Check sheet for the modelled part. Datum: model origin and axes. Units: mm. Face numbers are marked on the shaded views. A direction names the side the tool comes from. Round coordinates to 2 decimals unless told otherwise and drop trailing zeros. Order: outer loops, then holes, each group sorted by start corner. A loop starts at its lowest first (then second) coordinate and runs counter-clockwise, first axis right, second up. Notation, with made-up numbers: (24.25, 85.25) -> (63.25, 85.25) arc R12 cw to (63.25, 107.25) -> close; hole circle Ø6 at (32, 27.5). An arc over 180 degrees is marked (long way). Answer in a Markdown table with one row per item. Add a question column.
1. Sectioned sample at C-C, the plane x = 9.5. Record the boundary of the cut face in (y, z), then the cut area to 3 significant figures.
2. Depth check by flat-ended pin: P1, Ø0.8, axis at x = 13, z = 13, coming from the -Y side; P2, Ø0.5, axis at y = -13, z = 10, coming from the +X side; P3, Ø2.5, axis at x = -0.5, z = 10, coming from the +Y side. Enter the tip coordinate at first touch or a pass-through.
3. Draft check along Y on the marked faces 4, 5 and 6. Enter one of: +Y half, -Y half, draft (parallel to the pull), parting line (faces both ways), or undercut.
4. Sectioned sample at B-B, the plane y = 11.5. Record the boundary of the cut face in (x, z), then the cut area to 3 significant figures.
5. Material ranges on L1, parallel to X at y = 9, z = 17.5; L2, parallel to X at y = -5.5, z = 8.25; L3, parallel to X at y = 9.5, z = 11, recorded low to high. Write a range as from..to.
6. Sectioned sample at D-D, the plane x = 5. Record the boundary of the cut face in (y, z).
7. Access from +Z, -Z, +X, -X, +Y, -Y to the whole of each face (thin tool, end or side, straight path). Record for the marked faces 1, 2 and 3.
8. Sectioned sample at A-A, the plane x = 13. Record the boundary of the cut face in (y, z), then the cut area to 3 significant figures.
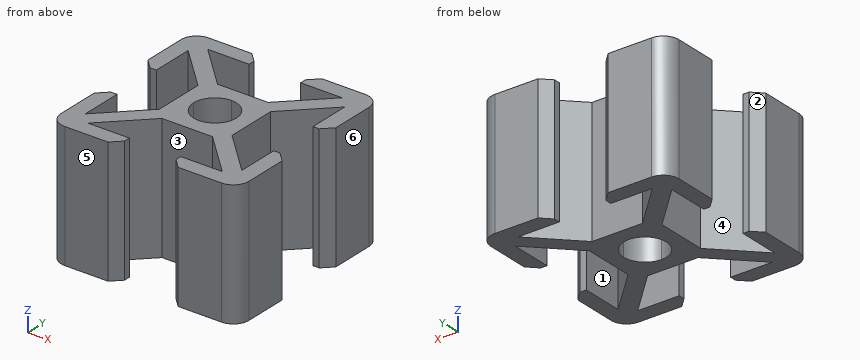
```python
from build123d import *

# Parameters (mm, degrees)
PAD_DEPTH            = 20
POLARPATTERN_COUNT   = 4
FILLET_R             = 2.5
CHAMFER_SIZE         = 1.5
BODY_PLACEMENT_ANGLE = 270


with BuildPart() as part:
    # Sketch → Pad (new body)
    with BuildSketch(Plane.XZ):
        with BuildLine():
            Line((0, 5.8), (4.032233, 5.8))
            Line((4.032233, 5.8), (10.732233, 12.5))
            Line((10.732233, 12.5), (4.1, 12.5))
            Line((4.1, 12.5), (4.1, 15))
            Line((4.1, 15), (15, 15))
            Line((15, 15), (15, 4.1))
            Line((15, 4.1), (12.5, 4.1))
            Line((12.5, 4.1), (12.5, 10.732233))
            Line((5.8, 4.032233), (12.5, 10.732233))
            Line((5.8, 4.032233), (5.8, 0))
            Line((3.4, 0), (5.8, 0))
            ThreePointArc((3.4, 0), (2.404163, 2.404163), (0, 3.4))
            Line((0, 5.8), (0, 3.4))
        make_face()
    pad = extrude(amount=PAD_DEPTH)

    # PolarPattern: Pad ×4 about axis
    polarpattern_axis = Axis((0, 0, 0), (0, -1, 0))
    for i in range(1, POLARPATTERN_COUNT):
        add(pad.rotate(polarpattern_axis, i * 360 / POLARPATTERN_COUNT))

    # Fillet
    fillet_edges = [part.edges().sort_by_distance(p)[0] for p in [
        (-15, -10, 15),
        (15, -10, 15),
        (15, -10, -15),
        (-15, -10, -15),
    ]]
    fillet(fillet_edges, radius=FILLET_R)

    # Chamfer
    chamfer_edges = [part.edges().sort_by_distance(p)[0] for p in [
        (4.1, -10, 15),
        (-4.1, -10, 15),
        (-15, -10, 4.1),
        (-15, -10, -4.1),
        (-4.1, -10, -15),
        (15, -10, -4.1),
        (4.1, -10, -15),
        (15, -10, 4.1),
    ]]
    chamfer(chamfer_edges, length=CHAMFER_SIZE)


with BuildPart() as part_1:
    # Body placement: moved
    add(part.part.rotate(Axis((0, 0, 0), (1, 0, 0)), BODY_PLACEMENT_ANGLE))


solid = part_1.part
```
Answer key:
| question | item | result |
|---|---|---|
| 1 | outline | (-15, 0) -> (-12.5, 0) -> (-12.5, 20) -> (-15, 20) -> close; (-11.27, 0) -> (-7.73, 0) -> (-7.73, 20) -> (-11.27, 20) -> close; (7.73, 0) -> (11.27, 0) -> (11.27, 20) -> (7.73, 20) -> close; (12.5, 0) -> (15, 0) -> (15, 20) -> (12.5, 20) -> close |
| 1 | area | 241 mm² |
| 2 | P1 | stops at y = -15 |
| 2 | P2 | stops at x = 14.99 |
| 2 | P3 | stops at y = 5.8 |
| 3 | face 4 | undercut |
| 3 | face 5 | -Y half |
| 3 | face 6 | draft |
| 4 | outline | (-15, 0) -> (-9.73, 0) -> (-9.73, 20) -> (-15, 20) -> close; (9.73, 0) -> (15, 0) -> (15, 20) -> (9.73, 20) -> close |
| 4 | area | 211 mm² |
| 5 | L1 | x = -15..-12.5, -10.77..-7.23, 7.23..10.77, 12.5..15 |
| 5 | L2 | x = -14.9..-12.5, -7.27..7.27, 12.5..14.9 |
| 5 | L3 | x = -15..-12.5, -11.27..-7.73, 7.73..11.27, 12.5..15 |
| 6 | outline | (-14.4, 0) -> (-12.5, 0) -> (-12.5, 20) -> (-14.4, 20) -> close; (-6.77, 0) -> (6.77, 0) -> (6.77, 20) -> (-6.77, 20) -> close; (12.5, 0) -> (14.4, 0) -> (14.4, 20) -> (12.5, 20) -> close |
| 7 | face 1 | +Z, -Z |
| 7 | face 2 | +Z, -Z, -X |
| 7 | face 3 | +Z, -Z, -Y |
| 8 | outline | (-14.95, 0) -> (-4.1, 0) -> (-4.1, 20) -> (-14.95, 20) -> close; (4.1, 0) -> (14.95, 0) -> (14.95, 20) -> (4.1, 20) -> close |
| 8 | area | 434 mm² |
